Geometry check sheet. Reference: the model listing, model coordinates, mm. Face numbers are marked on the shaded views. A direction names the side the tool comes from. Round coordinates to 2 decimals unless told otherwise and drop trailing zeros. Write each loop counter-clockwise with the first axis right and the second up, starting at its lowest first coordinate (ties: lowest second). Pieces come first, ordered by that corner, then holes. Notation, with made-up numbers: M 37.5,72 L 68.5,72 A35 ccw 68.5,107 Z; hole C -9,-13.5 d10. An arc over 180 degrees is marked long. Put each result on its own line as item: value. Start each with the question number.
(1) Section check A-A on y = 9. Record the cut outline in (x, z).
(2) Section check B-B on x = 53.5. Record the cut outline in (y, z).
(3) Gauge pin test, flat ends, axial feed: pin 1 (1 mm diameter, centred on x = 46, z = 7, fed in from +Y); pin 2 (8 mm diameter, centred on x = 15, y = 7.5, fed in from +Z); pin 3 (4 mm diameter, centred on x = 37, y = 38, fed in from +Z); pin 4 (2 mm diameter, centred on x = 5, z = 2.5, fed in from +Y). Record the tip position at first contact, or that the pin passes through.
(4) Material ranges on probe 1 along Y at (x, z) = (32.5, 1.5); probe 2 along Z at (x, y) = (27.5, 32); probe 3 along Y at (x, z) = (38, 4), recorded low to high.
(5) Tool access check on the marked faces 1, 2, 3 and 4. Record the directions out of +Z, -Z, +X, -X, +Y, -Y that give a thin tool (end or side, any length) a straight path to the whole face; none if there is none.
(6) Mould release check, pull along Y, two halves, no side actions. Record for the marked faces 5, 6, 7 and 8: pulls with the +Y half, pulls with the -Y half, needs draft (parallel to the pull), parting line crosses it, or undercut.
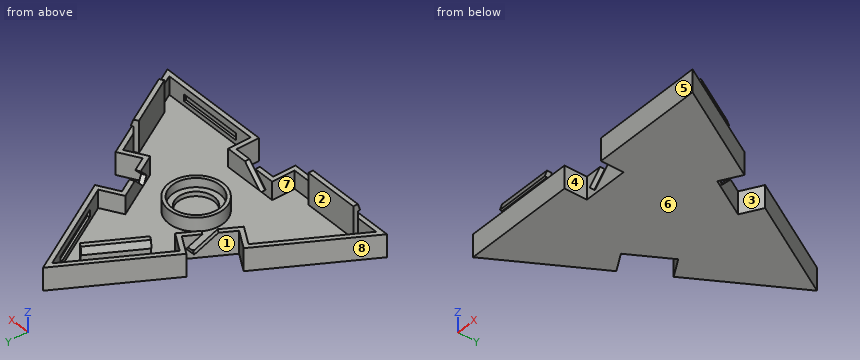
from build123d import *

# Parameters (mm, degrees)
F1_DEPTH     = 10
F2_W         = 10
F2_H         = 10
F3_DEPTH     = 5
F4_W         = 10
F4_H         = 10
F5_DEPTH     = 5
F6_W         = 10
F6_H         = 10
F7_DEPTH     = 5
F9_DEPTH     = 9
F10_DEPTH    = 5
F11_W        = 12.2679491924
F11_H        = 4
F11_H_2      = 3
F12_DEPTH    = 1
F13_W        = 12.2679491924
F13_H        = 4
F13_H_2      = 3
F14_DEPTH    = 1
F15_W        = 12.2679491924
F15_H        = 4
F15_H_2      = 3
F16_DEPTH    = 1
F17_W        = 12.2679491924
F17_H        = 1.5
F18_DEPTH    = 0.5
F19_T1_DEPTH = 20.0531322244
F20_W        = 12.2679491924
F20_H        = 1.5
F21_DEPTH    = 0.5
F22_T1_DEPTH = 20.0531322244
F23_W        = 12.2679491924
F23_H        = 1.5
F24_DEPTH    = 0.5
F25_T1_DEPTH = 20.0531322244
F26_W        = 14.2679491924
F26_H        = 1.5
F27_DEPTH    = 0.5
F28_W        = 14.2679491924
F28_H        = 1.5
F29_DEPTH    = 0.5
F30_W        = 14.2679491924
F30_H        = 1.5
F31_DEPTH    = 0.5
F32_R        = 6
F33_DEPTH    = 4
F34_R        = 5.25
F35_DEPTH    = 3
F36_R        = 4
F37_DEPTH    = 1
F39_DEPTH    = 1
F41_DEPTH    = 1
F43_DEPTH    = 1
F44_DEPTH    = 1


# Not quite as in the source:
# - a fillet or chamfer that OpenCascade refuses, or shapes differently, is made with other operations: its cross-section is extruded or revolved along the edge and cut away or added


with BuildPart() as f1:
    # F0 (on Top) → F1 (new body)
    with BuildSketch(Plane.XY):
        Polygon((30, 51.9615242271), (0, 0), (60, 0), align=None)
    extrude(amount=F1_DEPTH)

    # F2 (on face) → F3 (cut)
    with BuildSketch(Plane.XZ):
        with Locations((30, 5)):
            Rectangle(F2_W, F2_H)
    extrude(amount=-F3_DEPTH, mode=Mode.SUBTRACT)

    # F4 (on face) → F5 (cut)
    with BuildSketch(Plane(origin=(0, 0, 0), x_dir=(-0.5, -0.8660254038, 0), z_dir=(-0.8660254038, 0.5, 0))):
        with Locations((-30, 5)):
            Rectangle(F4_W, F4_H)
    extrude(amount=-F5_DEPTH, mode=Mode.SUBTRACT)

    # F6 (on face) → F7 (cut)
    with BuildSketch(Plane(origin=(45, 25.9807621135, 0), x_dir=(-0.5, 0.8660254038, 0), z_dir=(0.8660254038, 0.5, 0))):
        with Locations((0, 5)):
            Rectangle(F6_W, F6_H)
    extrude(amount=-F7_DEPTH, mode=Mode.SUBTRACT)

    # F8 (on face) → F9 (cut)
    with BuildSketch(Plane.XY.offset(10)):
        Polygon((18.8660254038, 30.6769145362), (23.1961524227, 28.1769145362), (17.1961524227, 17.7846096908), (12.8660254038, 20.2846096908), (1.7320508076, 1), (24, 1), (24, 6), (36, 6), (36, 1), (58.2679491924, 1), (47.1339745962, 20.2846096908), (42.8038475773, 17.7846096908), (36.8038475773, 28.1769145362), (41.1339745962, 30.6769145362), (30, 49.9615242271), align=None)
    extrude(amount=-F9_DEPTH, mode=Mode.SUBTRACT)

    # F10 (cut): a face of the model
    f10_faces = [f1.faces().sort_by_distance(p)[0] for p in [
        (35.7937253933, 2.5, 10),
    ]]
    extrude(f10_faces, amount=-F10_DEPTH, mode=Mode.SUBTRACT)

    # F11 (on face) → F12 (join)
    with BuildSketch(Plane(origin=(0.8660254038, -0.5, 0), x_dir=(0.5, 0.8660254038, 0), z_dir=(0.8660254038, -0.5, 0))):
        with Locations((47.1339745962, 3)):
            Rectangle(F11_W, F11_H)
        with Locations((47.1339745962, 6.5)):
            Rectangle(F11_W, F11_H_2)
    extrude(amount=F12_DEPTH)

    # F13 (on face) → F14 (join)
    with BuildSketch(Plane(origin=(0, 1, 0), x_dir=(-1, 0, 0), z_dir=(0, 1, 0))):
        with Locations((-12.8660254038, 3)):
            Rectangle(F13_W, F13_H)
        with Locations((-12.8660254038, 6.5)):
            Rectangle(F13_W, F13_H_2)
    extrude(amount=F14_DEPTH)

    # F15 (on face) → F16 (join)
    with BuildSketch(Plane(origin=(44.1339745962, 25.4807621135, 0), x_dir=(0.5, -0.8660254038, 0), z_dir=(-0.8660254038, -0.5, 0))):
        with Locations((17.1339745962, 3)):
            Rectangle(F15_W, F15_H)
        with Locations((17.1339745962, 6.5)):
            Rectangle(F15_W, F15_H_2)
    extrude(amount=F16_DEPTH)

    # F17 (on face) → F18 (join)
    with BuildSketch(Plane.XZ.offset(-1)):
        with Locations((12.8660254038, 7.25)):
            Rectangle(F17_W, F17_H)
    extrude(amount=F18_DEPTH)

    # F19: chamfer of 0.5 x 1.5 on 1 edges, made by hand

    # F19_s2 → F19_t1 (cut)
    with BuildSketch(Plane.YZ.offset(2.8394592916)):
        Polygon((0.5, 6.5), (1, 8), (0.5, 8), align=None)
    extrude(amount=F19_T1_DEPTH, mode=Mode.SUBTRACT)

    # F20 (on face) → F21 (join)
    with BuildSketch(Plane(origin=(44.1339745962, 25.4807621135, 0), x_dir=(-0.5, 0.8660254038, 0), z_dir=(0.8660254038, 0.5, 0))):
        with Locations((-17.1339745962, 7.25)):
            Rectangle(F20_W, F20_H)
    extrude(amount=F21_DEPTH)

    # F22: chamfer of 0.5 x 1.5 on 1 edges, made by hand

    # F22_s2 → F22_t1 (cut)
    with BuildSketch(Plane(origin=(3.553704242, -6.1551963022, 0), x_dir=(0, 0, 1), z_dir=(0.5, -0.8660254038, 0))):
        Polygon((6.5, -51.4615242271), (8, -50.9615242271), (8, -51.4615242271), align=None)
    extrude(amount=F22_T1_DEPTH, mode=Mode.SUBTRACT)

    # F23 (on face) → F24 (join)
    with BuildSketch(Plane(origin=(0.8660254038, -0.5, 0), x_dir=(-0.5, -0.8660254038, 0), z_dir=(-0.8660254038, 0.5, 0))):
        with Locations((-47.1339745962, 7.25)):
            Rectangle(F23_W, F23_H)
    extrude(amount=F24_DEPTH)

    # F25: chamfer of 0.5 x 1.5 on 1 edges, made by hand

    # F25_s2 → F25_t1 (cut)
    with BuildSketch(Plane(origin=(18.553704242, 32.1359584158, 0), x_dir=(0, 0, 1), z_dir=(0.5, 0.8660254038, 0))):
        Polygon((6.5, 0.5), (8, 1), (8, 0.5), align=None)
    extrude(amount=F25_T1_DEPTH, mode=Mode.SUBTRACT)

    # F26 (on face) → F27 (cut)
    with BuildSketch(Plane(origin=(44.1339745962, 25.4807621135, 0), x_dir=(0.5, -0.8660254038, 0), z_dir=(-0.8660254038, -0.5, 0))):
        with Locations((-17.1339745962, 2.75)):
            Rectangle(F26_W, F26_H)
    extrude(amount=-F27_DEPTH, mode=Mode.SUBTRACT)

    # F28 (on face) → F29 (cut)
    with BuildSketch(Plane(origin=(0, 1, 0), x_dir=(-1, 0, 0), z_dir=(0, 1, 0))):
        with Locations((-47.1339745962, 2.75)):
            Rectangle(F28_W, F28_H)
    extrude(amount=-F29_DEPTH, mode=Mode.SUBTRACT)

    # F30 (on face) → F31 (cut)
    with BuildSketch(Plane(origin=(0.8660254038, -0.5, 0), x_dir=(0.5, 0.8660254038, 0), z_dir=(0.8660254038, -0.5, 0))):
        with Locations((12.8660254038, 2.75)):
            Rectangle(F30_W, F30_H)
    extrude(amount=-F31_DEPTH, mode=Mode.SUBTRACT)

    # F32 (on face) → F33 (join)
    with BuildSketch(Plane.XY.offset(1)):
        with Locations((30, 18)):
            Circle(F32_R)
    extrude(amount=F33_DEPTH)

    # F34 (on face) → F35 (cut)
    with BuildSketch(Plane.XY.offset(5)):
        with Locations((30, 18)):
            Circle(F34_R)
    extrude(amount=-F35_DEPTH, mode=Mode.SUBTRACT)

    # F36 (on face) → F37 (cut)
    with BuildSketch(Plane.XY.offset(2)):
        with Locations((30, 18)):
            Circle(F36_R)
    extrude(amount=-F37_DEPTH, mode=Mode.SUBTRACT)

    # F38 (on face) → F39 (cut)
    with BuildSketch(Plane.XZ.offset(-5)):
        Polygon((25.7573593129, 2.1715728753), (27.1715728753, 0.7573593129), (31.4142135624, 5), (28.5857864376, 5), align=None)
    extrude(amount=-F39_DEPTH, mode=Mode.SUBTRACT)

    # F40 (on face) → F41 (cut)
    with BuildSketch(Plane(origin=(40.6698729811, 23.4807621135, 0), x_dir=(-0.5, 0.8660254038, 0), z_dir=(0.8660254038, 0.5, 0))):
        Polygon((-4.2426406871, 2.1715728753), (-2.8284271247, 0.7573593129), (1.4142135624, 5), (-1.4142135624, 5), align=None)
    extrude(amount=-F41_DEPTH, mode=Mode.SUBTRACT)

    # F42 (on face) → F43 (cut)
    with BuildSketch(Plane(origin=(4.3301270189, -2.5, 0), x_dir=(-0.5, -0.8660254038, 0), z_dir=(-0.8660254038, 0.5, 0))):
        Polygon((-34.2426406871, 2.1715728753), (-32.8284271247, 0.7573593129), (-28.5857864376, 5), (-31.4142135624, 5), align=None)
    extrude(amount=-F43_DEPTH, mode=Mode.SUBTRACT)

    # F44 (cut): a face of the model
    f44_faces = [f1.faces().sort_by_distance(p)[0] for p in [
        (24.1697056275, 18, 5),
    ]]
    extrude(f44_faces, amount=-F44_DEPTH, mode=Mode.SUBTRACT)


solid = f1.part
Answers follow:
1. outline: M 5.2,0 L 54.8,0 L 54.8,5 L 53.65,5 L 53.65,6.5 L 54.23,6.5 L 53.65,8 L 52.49,8 L 52.49,1 L 6.35,1 L 6.35,2 L 5.77,2 L 5.77,3.5 L 6.35,3.5 L 6.35,5 L 5.2,5 Z
2. outline: M 0,0 L 11.26,0 L 11.26,5 L 9.26,5 L 9.26,6.5 L 10.26,6.5 L 9.26,8 L 7.26,8 L 7.26,1 L 1,1 L 1,2 L 0.5,2 L 0.5,3.5 L 1,3.5 L 1,5 L 0,5 Z
3. pin 1: passes through
3. pin 2: stops at z = 1
3. pin 3: stops at z = 5
3. pin 4: stops at y = 10.39
4. probe 1: y = 5 to 6, 12.55 to 14.88, 21.12 to 23.45, 45.63 to 47.63
4. probe 2: z = 0 to 1
4. probe 3: y = 0 to 1, 26.11 to 28.87, 36.11 to 38.11
5. face 1: +Z, -Z
5. face 2: +Z
5. face 3: +Z, -Z, +X
5. face 4: +Z, -Z, -Y
6. face 5: pulls with the -Y half
6. face 6: needs draft
6. face 7: undercut
6. face 8: pulls with the +Y half
